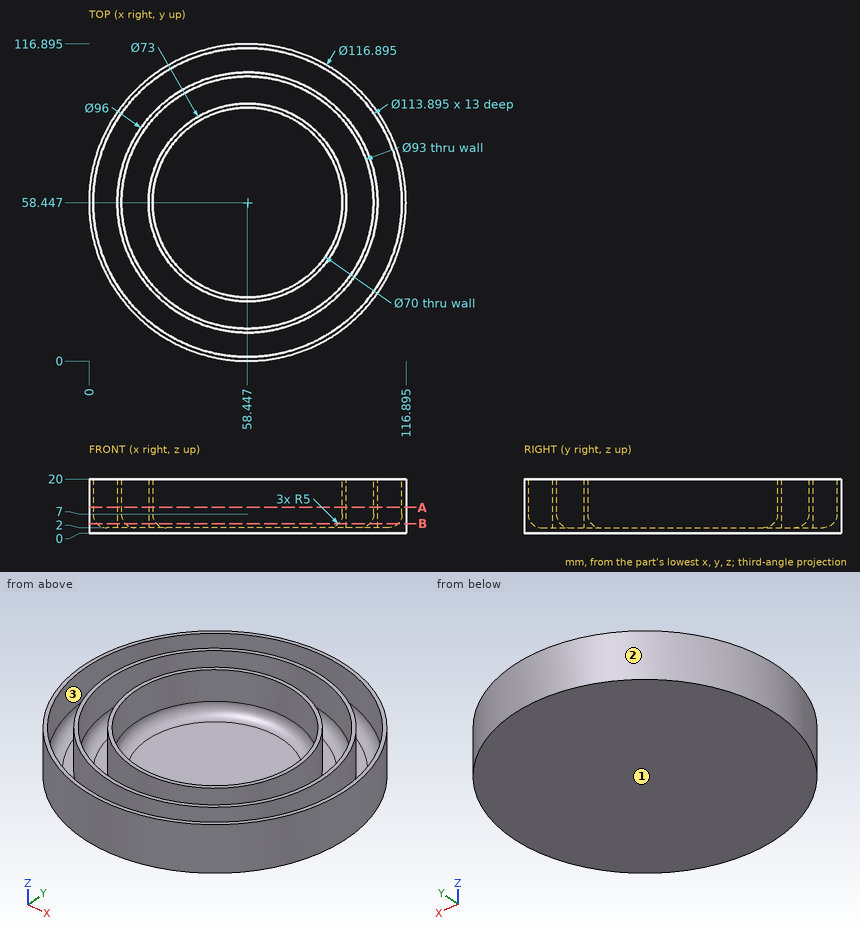
Here's the drawing with two shaded views (mm, measured from the low corner). I have some questions. Coordinates: 2 decimals unless noted, no trailing zeros. Loops run counter-clockwise (first coordinate to the right, second up) from the corner with the lowest first, then second, coordinate; pieces in that order, holes last. Notation, with made-up numbers: M 51,55 L 102,55 A20 cw 102,75 Z; hole C 35.25,38 d4. An arc over 180 degrees is marked long. Answer as CSV lines item,"result". Start each with the question number.
1. Suppose I cut it at B-B, the plane z = 3.5. List the corners of the cut face in (x, y) for me (1 decimal).
2. Suppose I cut it at A-A, the plane z = 9.5. List the corners of the cut face in (x, y) for me (1 decimal).
3. Thinking about a two-plate mould opening in Y: for the marked faces 1, 2 and 3, which applies, +Y half, -Y half, draft (parallel to the pull), parting line (faces both ways), or undercut?
4. For pin 1 Ø4 at (x, y) = (55, 32) entering from +Z; pin 2 Ø2 at (x, y) = (93, 96) entering from -Z; pin 3 Ø1 at (x, z) = (25.5, 11) entering from -Y (1 decimal); pin 4 Ø1.5 at (y, z) = (37, 7) entering from -X, each with a flat end and sliding along its axis, tell me the tip position at first contact or that it passes through.
5. If I drill on probe 1 along Y at (x, z) = (16, 10.25) (1 decimal); probe 2 along X at (y, z) = (82, 9) (1 decimal); probe 3 along X at (y, z) = (49, 15) (1 decimal), over which ranges is the centre line in solid material (lowest first)? Write a range as [from, to].
Output:
1,outline,"C 58.4,58.4 d116.9; C 58.4,58.4 d96; C 58.4,58.4 d73; hole C 58.4,58.4 d111; hole C 58.4,58.4 d90.1; hole C 58.4,58.4 d67.1"
2,outline,"C 58.4,58.4 d116.9; C 58.4,58.4 d96; C 58.4,58.4 d73; hole C 58.4,58.4 d113.9; hole C 58.4,58.4 d93; hole C 58.4,58.4 d70"
3,face 1,"draft"
3,face 2,"parting line"
3,face 3,"undercut"
4,pin 1,"stops at z = 2"
4,pin 2,"stops at z = 0"
4,pin 3,"stops at y = 9.8"
4,pin 4,"stops at x = 3.79"
5,probe 1,"y = [18.3, 20.5], [36, 39.5], [77.4, 80.9], [96.4, 98.6]"
5,probe 2,"x = [5, 6.6], [16.6, 18.4], [30.6, 32.6], [84.3, 86.3], [98.5, 100.3], [110.3, 111.9]"
5,probe 3,"x = [0.8, 2.3], [11.4, 12.9], [23.2, 24.7], [92.1, 93.7], [104, 105.5], [114.6, 116.1]"
